from build123d import *

# Parameters (mm, degrees)
F1_DEPTH = 63.5
F2_DEPTH = 25.4
F3_DEPTH = 7.9375
F5_R     = 6.35


with BuildPart() as f1:
    # F0 (on Front) → F1 (new body, symmetric)
    with BuildSketch(Plane.XZ):
        Polygon((41.275, -9.525), (41.275, 9.525), (22.225, 9.525), (-41.275, 9.525), (-41.275, -9.525), align=None)
    extrude(amount=F1_DEPTH, both=True)

    # F0 (on Front) → F2 (join, symmetric)
    with BuildSketch(Plane.XZ):
        with BuildLine():
            Line((22.225, 9.525), (41.275, 9.525))
            Line((41.275, 9.525), (41.275, 27.0002))
            ThreePointArc((41.275, 27.0002), (45.92468, 38.22552), (57.15, 42.8752))
            Line((57.15, 42.8752), (60.325, 42.8752))
            Line((60.325, 42.8752), (60.325, 61.9252))
            Line((60.325, 61.9252), (57.15, 61.9252))
            ThreePointArc((57.15, 61.9252), (32.454296, 51.695904), (22.225, 27.0002))
            Line((22.225, 27.0002), (22.225, 9.525))
        make_face()
    extrude(amount=F2_DEPTH, both=True)

    # F0 (on Front) → F3 (join, symmetric)
    with BuildSketch(Plane.XZ):
        with BuildLine():
            Line((-41.275, 9.525), (22.225, 9.525))
            Line((22.225, 9.525), (22.225, 27.0002))
            ThreePointArc((22.225, 27.0002), (32.454296, 51.695904), (57.15, 61.9252))
            add(Edge.make_bspline(
                [(-41.275, 9.525), (-42.136356, 39.629813), (22.141983, 62.799598), (57.15, 61.9252)],
                knots=[0, 0, 0, 0, 111.504536, 111.504536, 111.504536, 111.504536], degree=3))
        make_face()
    extrude(amount=F3_DEPTH, both=True)

    # F0 (on Front) → F4 (revolve)
    with BuildSketch(Plane.XZ):
        Polygon((82.928714, 61.9252), (82.928714, 42.8752), (82.928714, 38.1), (111.125, 38.1), (111.125, 66.675), (82.928714, 66.675), align=None)
    revolve(axis=Axis((82.928714, 0, 52.3875), (0, 0, 1)))

    # F5
    f5_edges = [f1.edges().sort_by_distance(p)[0] for p in [
        (41.275, -63.5, 0),
        (-41.275, -63.5, 0),
        (41.275, 63.5, 0),
        (-41.275, 63.5, 0),
    ]]
    fillet(f5_edges, radius=F5_R)


solid = f1.part
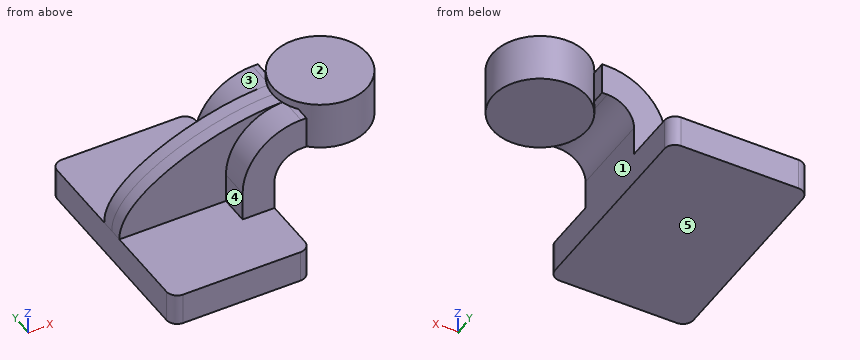
Here's how the part is built. I have some questions about the finished solid (model axes, mm). Face numbers are marked on the shaded views. A direction names the side the tool comes from. Give positions to 0.01 mm unless a question says otherwise; leave off trailing zeros. Order: outer loops, then holes, each group sorted by start corner. A loop starts at its lowest first (then second) coordinate and runs counter-clockwise, first axis right, second up. Notation, with made-up numbers: M -11.75,3.5 L 24.25,3.5 A20 cw 24.25,21.5 Z; hole C 11.5,7 d1. An arc over 180 degrees is marked long. Answer as a JSON object with one key per item and string values. Group by question number.
1) Suppose I cut it at A-A, the plane z = -0.5. Write out the boundary of the cut face in (x, y) (3 decimals), plus the area to 3 significant figures.
2) Suppose I cut it at B-B, the plane y = 48. Write out the boundary of the cut face in (x, z) (3 decimals), plus the area to 3 significant figures.
3) I'm going to push flat-ended pins straight in: pin 1 Ø15 at (y, z) = (24.5, 0) entering from -X (3 decimals); pin 2 Ø8 at (x, z) = (38, 25.5) entering from -Y; pin 3 Ø14 at (y, z) = (-18.5, 21) entering from -X (3 decimals); pin 4 Ø12 at (x, z) = (40.5, 7.5) entering from +Y. Where does each tip first touch, or does it pass through?
4) Suppose I cut it at C-C, the plane x = 91. Write out the boundary of the cut face in (y, z) (3 decimals), plus the area to 3 significant figures.
5) On a 3-axis mill with a long thin cutter (end or side, diameter ignored), from which of +Z, -Z, +X, -X, +Y, -Y can I reach the whole of each face in a straight line? I mean the marked faces 1, 2, 3, 4 and 5. Say none if no direction works.
6) Please list where these lines run through material, in increasing order: L1, parallel to Z at x = -26, y = -43 (3 decimals); L2, parallel to X at y = -26, z = 7 (3 decimals); L3, parallel to Y at x = 10, z = 18.5. Write a range as [from, to].
Results found:
{
 "1": {"outline": "M -41.275,-57.15 A6.35 ccw -34.925,-63.5 L 34.925,-63.5 A6.35 ccw 41.275,-57.15 L 41.275,57.15 A6.35 ccw 34.925,63.5 L -34.925,63.5 A6.35 ccw -41.275,57.15 Z", "area": "10,400 mm²"},
 "2": {"outline": "M -41.275,-9.525 L 41.275,-9.525 L 41.275,9.525 L -41.275,9.525 Z", "area": "1,570 mm²"},
 "3": {"pin 1": "x = -41.275", "pin 2": "y = -25.4", "pin 3": "x = 22.225", "pin 4": "y = 63.5"},
 "4": {"outline": "M -27.016,38.1 L 27.016,38.1 L 27.016,66.675 L -27.016,66.675 Z", "area": "1,540 mm²"},
 "5": {"face 1": "-Z, +X, +Y, -Y", "face 2": "+Z, +X, -X, +Y, -Y", "face 3": "+Z, -X, +Y", "face 4": "+Z, -X, -Y", "face 5": "-Z, +X, -X, +Y, -Y"},
 "6": {"L1": "[-9.525, 9.525]", "L2": "[-41.275, 41.275]", "L3": "[-7.94, 7.94]"}
}
